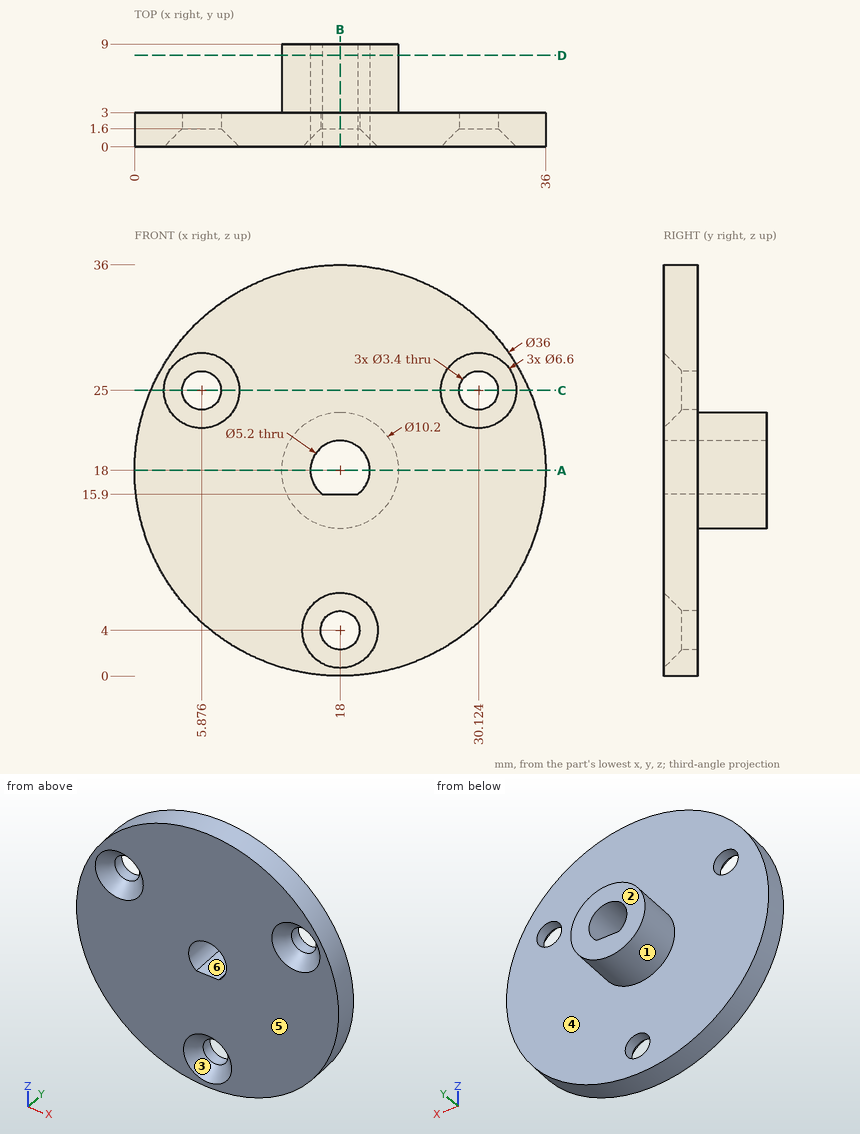
Geometry check sheet. Reference: drawing and pictorial views, mm from the part's lowest x, y, z. A direction names the side the tool comes from. Give positions to 0.01 mm unless a question says otherwise; leave off trailing zeros. Loops run counter-clockwise (first coordinate to the right, second up) from the corner with the lowest first, then second, coordinate; pieces in that order, holes last.
1. Section check D-D, the plane y = 8. Enter the section's corners in (x, z).
2. Set-up check for the marked faces 4, 5 and 6: record each of +Z, -Z, +X, -X, +Y, -Y from which the full face is reachable in a straight line by a thin tool's end or side.
3. Thickness scan on line 1 (X direction, y = 3.5, z = 18); line 2 (X direction, y = 2.35, z = 25) (1 decimal); line 3 (Y direction, x = 24, z = 17). Record the ranges inside material, lowest first.
4. Mould release check, pull along Z, two halves, no side actions. Record for the marked faces 1, 2 and 3: released by +Z, released by -Z, zero draft, split by the parting line, or undercut.
5. Section check B-B, the plane x = 18. Enter the section's corners in (y, z).
6. Section check A-A, the plane z = 18. Enter the section's corners in (x, y), then the cut area to 3 significant figures.
7. Go/stop test with flat-tipped pins: pin 1 Ø2.5 at (x, y) = (17.5, 3.5) entering from +Z; pin 2 Ø4 at (x, z) = (5.88, 25) entering from -Y (1 decimal); pin 3 Ø2 at (x, y) = (16, 7) entering from -Z; pin 4 Ø6 at (x, z) = (28.5, 30.5) entering from +Y. Record where each tip stops, or that it passes through.
8. Section check C-C, the plane z = 25. Enter the section's corners in (x, y) (1 decimal).
Geometry says:
1. outline: circle Ø10.2 at (18, 18); hole (16.47, 15.9) - (19.53, 15.9) arc R2.6 ccw (long way) to start
2. face 4: +Y
2. face 5: +Z, -Z, +X, -X, -Y
2. face 6: +Y, -Y
3. line 1: x = 12.9 to 15.4, 20.6 to 23.1
3. line 2: x = 1.4 to 4.2, 7.6 to 28.4, 31.8 to 34.6
3. line 3: y = 0 to 3
4. face 1: split by the parting line
4. face 2: zero draft
4. face 3: undercut
5. outline: (0, 0) - (3, 0) - (3, 2.3) - (1.6, 2.3) - (0, 0.7) - close; (0, 7.3) - (1.6, 5.7) - (3, 5.7) - (3, 12.9) - (9, 12.9) - (9, 15.9) - (0, 15.9) - close; (0, 20.6) - (9, 20.6) - (9, 23.1) - (3, 23.1) - (3, 36) - (0, 36) - close
6. outline: (0, 0) - (15.4, 0) - (15.4, 9) - (12.9, 9) - (12.9, 3) - (0, 3) - close; (20.6, 0) - (36, 0) - (36, 3) - (23.1, 3) - (23.1, 9) - (20.6, 9) - close
6. area: 122 mm2
7. pin 1: stops at z = 36
7. pin 2: stops at y = 1.3
7. pin 3: stops at z = 13
7. pin 4: stops at y = 3
8. outline: (1.4, 0) - (2.6, 0) - (4.2, 1.6) - (4.2, 3) - (1.4, 3) - close; (7.6, 1.6) - (9.2, 0) - (26.8, 0) - (28.4, 1.6) - (28.4, 3) - (7.6, 3) - close; (31.8, 1.6) - (33.4, 0) - (34.6, 0) - (34.6, 3) - (31.8, 3) - close
